Verification items for the finished model (mm, model axes). A direction names the side the tool comes from. Give positions to 0.01 mm unless a question says otherwise; leave off trailing zeros. Loops run counter-clockwise (first coordinate to the right, second up) from the corner with the lowest first, then second, coordinate; pieces in that order, holes last. Notation, with made-up numbers: (-13, 45.25) - (30, 45.25) arc R34 cw to (30, 81.25) - close; hole circle Ø1 at (-33.75, 70.25). An arc over 180 degrees is marked (long way). One line per item, written item: value. Start each with the question number.
1. Gauge pin test, flat ends, axial feed: pin 1 (5 mm diameter, centred on x = -511, y = 69, fed in from +Z); pin 2 (5.5 mm diameter, centred on x = -636.5, z = 126.5, fed in from -Y); pin 3 (2.5 mm diameter, centred on y = 168, z = 96, fed in from +X). Record the tip position at first contact, or that the pin passes through.
2. Sectioned sample at A-A (y = 140.5). Record the cut outline in (x, z).
3. Mould release check, pull along Y, two halves, no side actions. Record for faces 5 (the flat face through (-642, 9.123, 91)), 6 (the flat face through (-553, 176.823, 82)), 7 (the flat face through (-469.698, 86, 4)), 8 (the flat face through (-556, 86, -10)): pulls with the +Y half, pulls with the -Y half, needs draft (parallel to the pull), parting line crosses it, or undercut.
4. Access from +Z, -Z, +X, -X, +Y, -Y to the whole of each face (thin tool, end or side, straight path). Record for faces 1 (the flat face through (-554, -3.177, 4)), 2 (the flat face through (-644.698, 83, 85)), 3 (the flat face through (-468, 44, 7.5)), 4 (the flat face through (-476.998, 174, 91)).
5. Sectioned sample at B-B (z = 126). Record the cut outline in (x, y), plus the area to 3 significant figures.
6. Scan lines: L1, parallel to X at y = 15.5, z = 6.5; L2, parallel to Y at x = -515, z = 71; L3, parallel to Z at x = -615.5, y = 129. Record each from-to range of solid material in increasing order. Write a range as [from, to].
from build123d import *

# Parameters (mm, degrees)
CROQUIS1_W              = 180
CROQUIS1_H              = 185
SALIENTE_EXTRUIR1_DEPTH = 10
SALIENTE_EXTRUIR2_DEPTH = 7.5
SALIENTE_EXTRUIR3_DEPTH = 170
SALIENTE_EXTRUIR4_DEPTH = 177.5


with BuildPart() as part:
    # Croquis1 → Saliente-Extruir1 (new body)
    with BuildSketch(Plane.XY):
        with Locations((-554.698083647, 84.323121588)):
            Rectangle(CROQUIS1_W, CROQUIS1_H)
    extrude(amount=-SALIENTE_EXTRUIR1_DEPTH)

    # Croquis1<3> → Saliente-Extruir2 (add)
    with BuildSketch(Plane.XY):
        Polygon((-464.698083647, 176.823121588), (-476.998083647, 176.823121588), (-476.998083647, 171.823121588), (-469.698083647, 171.823121588), (-469.698083647, -3.176878412), (-639.698083647, -3.176878412), (-639.698083647, 9.123121588), (-644.698083647, 9.123121588), (-644.698083647, -8.176878412), (-464.698083647, -8.176878412), align=None)
    extrude(amount=SALIENTE_EXTRUIR2_DEPTH)

    # Croquis1<5> → Saliente-Extruir3 (add)
    with BuildSketch(Plane.XY):
        Polygon((-484.498083647, 166.823121588), (-484.498083647, 171.823121588), (-639.698083647, 171.823121588), (-639.698083647, 16.623121588), (-634.698083647, 16.623121588), (-634.698083647, 166.823121588), align=None)
    extrude(amount=SALIENTE_EXTRUIR3_DEPTH)

    # Croquis1<6> → Saliente-Extruir4 (add)
    with BuildSketch(Plane.XY):
        Polygon((-476.998083647, 171.823121588), (-476.998083647, 176.823121588), (-644.698083647, 176.823121588), (-644.698083647, 9.123121588), (-639.698083647, 9.123121588), (-639.698083647, 16.623121588), (-639.698083647, 171.823121588), (-484.498083647, 171.823121588), align=None)
    extrude(amount=SALIENTE_EXTRUIR4_DEPTH)


solid = part.part
Results are:
1. pin 1: stops at z = 0
1. pin 2: stops at y = 16.62
1. pin 3: stops at x = -484.5
2. outline: (-644.7, -10) - (-464.7, -10) - (-464.7, 7.5) - (-469.7, 7.5) - (-469.7, 0) - (-634.7, 0) - (-634.7, 170) - (-639.7, 170) - (-639.7, 177.5) - (-644.7, 177.5) - close
3. face 5: pulls with the -Y half
3. face 6: pulls with the +Y half
3. face 7: undercut
3. face 8: needs draft
4. face 1: +Z
4. face 2: +Z, -Z, -X, +Y, -Y
4. face 3: +Z, +X, -Y
4. face 4: +Z, +X, +Y, -Y
5. outline: (-644.7, 9.12) - (-639.7, 9.12) - (-639.7, 16.62) - (-634.7, 16.62) - (-634.7, 166.82) - (-484.5, 166.82) - (-484.5, 171.82) - (-477, 171.82) - (-477, 176.82) - (-644.7, 176.82) - close
5. area: 3,180 mm^2
6. L1: x = [-644.7, -639.7], [-469.7, -464.7]
6. L2: y = [166.82, 176.82]
6. L3: z = [-10, 0]
